Verification items for the finished model (mm, model axes). Give positions to 0.01 mm unless a question says otherwise; leave off trailing zeros. Loops run counter-clockwise (first coordinate to the right, second up) from the corner with the lowest first, then second, coordinate; pieces in that order, holes last. Notation, with made-up numbers: (4.25, -25.5) - (50.25, -25.5) arc R17 cw to (50.25, -3.5) - close; hole circle Ø1 at (-7, 10). An arc over 180 degrees is marked (long way). Use one line per item in the form item = value.
```python
from build123d import *

# Parameters (mm, degrees)
F1_DEPTH = 44.45
F2_R     = 3.175


with BuildPart() as f1:
    # F0 (on Front) → F1 (new body)
    with BuildSketch(Plane.XZ):
        with BuildLine():
            ThreePointArc((25.4, 53.975), (20.75032, 65.20032), (9.525, 69.85))
            Line((9.525, 69.85), (-9.525, 69.85))
            ThreePointArc((-9.525, 69.85), (-20.75032, 65.20032), (-25.4, 53.975))
            Line((-25.4, 53.975), (-25.4, -53.975))
            ThreePointArc((-25.4, -53.975), (-20.75032, -65.20032), (-9.525, -69.85))
            Line((-9.525, -69.85), (9.525, -69.85))
            ThreePointArc((9.525, -69.85), (20.75032, -65.20032), (25.4, -53.975))
            Line((25.4, -53.975), (25.4, 53.975))
        make_face()
    extrude(amount=F1_DEPTH)

    # F2
    f2_edges = [f1.edges().sort_by_distance(p)[0] for p in [
        (20.75032, -44.45, 65.20032),
        (0, -44.45, 69.85),
        (-20.75032, -44.45, 65.20032),
        (25.4, -44.45, 0),
        (20.75032, -44.45, -65.20032),
        (0, -44.45, -69.85),
        (-20.75032, -44.45, -65.20032),
        (-25.4, -44.45, 0),
        (20.75032, 0, 65.20032),
        (25.4, 0, 0),
        (20.75032, 0, -65.20032),
        (0, 0, 69.85),
        (-20.75032, 0, 65.20032),
        (0, 0, -69.85),
        (-20.75032, 0, -65.20032),
        (-25.4, 0, 0),
    ]]
    fillet(f2_edges, radius=F2_R)


solid = f1.part
```
1. Depth check by flat-ended pin: pin 1 Ø1.5 at (x, y) = (-11.5, -36) entering from +Z; pin 2 Ø5 at (x, y) = (20, -25) entering from -Z. Enter the tip coordinate at first touch or a pass-through.
Result set:
pin_1 = 69.8
pin_2 = -67.7
2. Draft check along Y on faces 1 (the flat face through (0, 0, 1)), 2 (the cylindrical face through (-20.87, -21.96, -65.08)), 3 (the cylindrical face through (24.49, -43.5, 0.76)). Enter one of: released by +Y, released by -Y, zero draft, split by the parting line, or undercut.
Result set:
face_1 = released by +Y
face_2 = zero draft
face_3 = released by -Y
3. Section check A-A, the plane y = -21.5. Record the cut outline in (x, z) (3 decimals).
Result set:
outline = (-25.4, -53.975) arc R15.875 ccw to (-9.525, -69.85) - (9.525, -69.85) arc R15.875 ccw to (25.4, -53.975) - (25.4, 53.975) arc R15.875 ccw to (9.525, 69.85) - (-9.525, 69.85) arc R15.875 ccw to (-25.4, 53.975) - close
4. Scan lines: probe 1 along Z at (x, y) = (-8, -1.5); probe 2 along Z at (x, y) = (-22, -24); probe 3 along X at (y, z) = (-42, 35.5). Record each from-to range of solid material in increasing order.
Result set:
probe_1 = -69.37 to 69.37
probe_2 = -63.79 to 63.79
probe_3 = -25.32 to 25.32
